from build123d import *

# Parameters (mm, degrees)
BOSS_EXTRUDE1_DEPTH          = 6.35
SKETCH2_W                    = 127
SKETCH2_H                    = 19.05
CUT_EXTRUDE1_DEPTH           = 195.543611155
SKETCH3_W                    = 86.864773719
SKETCH3_H                    = 114.3
BOSS_EXTRUDE2_DEPTH          = 6.35
SKETCH4_W                    = 6.35
SKETCH4_H                    = 9.525
SKETCH4_H_2                  = 44.45
SKETCH4_H_3                  = 15.875
CUT_EXTRUDE2_DEPTH           = 253.93516292
SKETCH5_W                    = 19.05
SKETCH5_H                    = 6.35
BOSS_EXTRUDE3_DEPTH          = 6.35
BOSS_EXTRUDE4_DEPTH          = 6.35
LPATTERN1_COUNT              = 2
LPATTERN1_PITCH              = 50.8
F_10_0_1935_DIAMETER_HOLE1_D = 4.9149
F_10_0_1935_DIAMETER_HOLE2_D = 4.9149
F_10_0_1935_DIAMETER_HOLE3_D = 4.9149


with BuildPart() as part:
    # Sketch1 → Boss-Extrude1 (new body)
    with BuildSketch(Plane.XY):
        Polygon((86.864773719, 57.15), (185.851477372, 0), (86.864773719, 0), (0, 0), (0, 57.15), align=None)
    extrude(amount=BOSS_EXTRUDE1_DEPTH)

    # Sketch2 → Cut-Extrude1 (cut, through all)
    with BuildSketch(Plane.XY.offset(6.35)):
        with Locations((69.85, 9.525)):
            Rectangle(SKETCH2_W, SKETCH2_H)
    extrude(amount=-CUT_EXTRUDE1_DEPTH, mode=Mode.SUBTRACT)

    # Sketch3 → Boss-Extrude2 (add)
    with BuildSketch(Plane.XY.offset(6.35)):
        with Locations((43.432386859, 114.3)):
            Rectangle(SKETCH3_W, SKETCH3_H)
    extrude(amount=-BOSS_EXTRUDE2_DEPTH)

    # Sketch4 → Cut-Extrude2 (cut, through all)
    with BuildSketch(Plane.XY.offset(6.35)):
        with Locations((3.175, 4.7625)):
            Rectangle(SKETCH4_W, SKETCH4_H)
        with Locations((3.175, 50.8)):
            Rectangle(SKETCH4_W, SKETCH4_H_2)
        with Locations((3.175, 114.3)):
            Rectangle(SKETCH4_W, SKETCH4_H_2)
        with Locations((3.175, 163.5125)):
            Rectangle(SKETCH4_W, SKETCH4_H_3)
    extrude(amount=-CUT_EXTRUDE2_DEPTH, mode=Mode.SUBTRACT)

    # Sketch5 → Boss-Extrude3 (add)
    with BuildSketch(Plane.XY.offset(6.35)):
        with Locations((158.75, -3.175)):
            Rectangle(SKETCH5_W, SKETCH5_H)
    extrude(amount=-BOSS_EXTRUDE3_DEPTH)

    # Sketch6 → Boss-Extrude4 (add)
    with BuildSketch(Plane.XY.offset(6.35)):
        Polygon((108.861818976, 44.45), (125.359602918, 34.925), (128.534602918, 40.424261314), (112.036818976, 49.949261314), align=None)
    boss_extrude4 = extrude(amount=-BOSS_EXTRUDE4_DEPTH)

    # LPattern1: Boss-Extrude4 ×2
    with Locations(*[Vector(0.8660254037844415, -0.49999999999999517, 0) * (i * LPATTERN1_PITCH) for i in range(1, LPATTERN1_COUNT)]):
        add(boss_extrude4)

    # #10 (0.1935) Diameter Hole1 (through all)
    with Locations(Plane.XY.offset(6.35)):
        with Locations((3.175, 146.05), (3.175, 82.55), (3.175, 19.05)):
            Hole(F_10_0_1935_DIAMETER_HOLE1_D / 2)

    # #10 (0.1935) Diameter Hole2 (through all)
    with Locations(Plane.XY.offset(6.35)):
        with Locations((118.698210947, 42.437130657), (162.692301459, 17.037130657), (158.75, -3.175)):
            Hole(F_10_0_1935_DIAMETER_HOLE2_D / 2)

    # #10 (0.1935) Diameter Hole3 (through all)
    with Locations(Plane.XY.offset(6.35)):
        with Locations((146.05, 6.35), (165.1, 6.35)):
            Hole(F_10_0_1935_DIAMETER_HOLE3_D / 2)


solid = part.part
Verification items for the finished model (mm, model axes). A direction names the side the tool comes from. Round coordinates to 2 decimals unless told otherwise and drop trailing zeros. Write each loop counter-clockwise with the first axis right and the second up, starting at its lowest first coordinate (ties: lowest second). Pieces come first, ordered by that corner, then holes.
(1) Section check D-D (y = 113). Enter the section's corners in (x, z).
Returned:
outline: (6.35, 0) - (86.86, 0) - (86.86, 6.35) - (6.35, 6.35) - close
(2) Material ranges on line 1 (X direction, y = 146, z = 5.75); line 2 (X direction, y = 8, z = 3.5); line 3 (X direction, y = 5.5, z = 4.75), recorded low to high.
Returned:
line 1: x = 0 to 0.72, 5.63 to 86.86
line 2: x = 133.35 to 144.23, 147.87 to 163.28, 166.92 to 172
line 3: x = 133.35 to 143.74, 148.36 to 162.79, 167.41 to 176.33
(3) Section check C-C (x = 58). Enter the section's corners in (y, z), plus the area to 3 significant figures.
Returned:
outline: (19.05, 0) - (171.45, 0) - (171.45, 6.35) - (19.05, 6.35) - close
area: 968 mm2
(4) Depth check by flat-ended pin: pin 1 Ø6.5 at (x, y) = (3.175, 19.05) entering from -Z; pin 2 Ø1.9 at (y, z) = (130.5, 2) entering from +X; pin 3 Ø3 at (x, z) = (3, 3.5) entering from -Y (3 decimals); pin 4 Ø1 at (y, z) = (63, 4.5) entering from -X. Enter the tip coordinate at first touch or a pass-through.
Returned:
pin 1: stops at z = 0
pin 2: stops at x = 86.86
pin 3: stops at y = 9.525
pin 4: stops at x = 6.35
(5) Section check B-B (y = 6.35). Enter the section's corners in (x, z), plus the area to 3 significant figures.
Returned:
outline: (133.35, 0) - (143.59, 0) - (143.59, 6.35) - (133.35, 6.35) - close; (148.51, 0) - (162.64, 0) - (162.64, 6.35) - (148.51, 6.35) - close; (167.56, 0) - (174.85, 0) - (174.85, 6.35) - (167.56, 6.35) - close
area: 201 mm2
(6) Mould release check, pull along Y, two halves, no side actions. Record for faces 1 (the cylindrical face through (3.71, 16.65, 3.13)), 2 (the flat face through (0, 19, 3)), 3 (the flat face through (3, 155.575, 3)), 4 (the flat face through (159, -6.35, 3)): pulls with the +Y half, pulls with the -Y half, needs draft (parallel to the pull), parting line crosses it, or undercut.
Returned:
face 1: undercut
face 2: needs draft
face 3: pulls with the +Y half
face 4: pulls with the -Y half
(7) Section check A-A (y = 82.55). Enter the section's corners in (x, z), plus the area to 3 significant figures.
Returned:
outline: (0, 0) - (0.72, 0) - (0.72, 6.35) - (0, 6.35) - close; (5.63, 0) - (86.86, 0) - (86.86, 6.35) - (5.63, 6.35) - close
area: 520 mm2
(8) Access from +Z, -Z, +X, -X, +Y, -Y to the whole of each face (thin tool, end or side, straight path). Record for faces 5 (the flat face through (133.35, 9, 3)), 6 (the flat face through (177, 0, 3)), 7 (the flat face through (6.35, 50, 3)), 8 (the flat face through (86.865, 113, 3)).
Returned:
face 5: +Z, -Z, -Y
face 6: +Z, -Z, +X, -Y
face 7: +Z, -Z, -X
face 8: +Z, -Z, +X, +Y
